```python
from build123d import *

# Parameters (mm, degrees)
F0_R     = 51.5
F1_DEPTH = 20
F2_R     = 49.925
F3_DEPTH = 17
F4_R     = 15.25
F5_DEPTH = 25
F8_R     = 10
F9_R     = 2


with BuildPart() as f1:
    # F0 (on Top) → F1 (new body)
    with BuildSketch(Plane.XY):
        Circle(F0_R)
    extrude(amount=F1_DEPTH)

    # F2 (on face) → F3 (cut)
    with BuildSketch(Plane.XY.offset(20)):
        Circle(F2_R)
    extrude(amount=-F3_DEPTH, mode=Mode.SUBTRACT)

    # F4 (on face) → F5 (cut)
    with BuildSketch(Plane(origin=(0, 0, 0), x_dir=(1, 0, 0), z_dir=(0, 0, -1))):
        Circle(F4_R)
    extrude(amount=-F5_DEPTH, mode=Mode.SUBTRACT)

    # F7: sweep along a path in F7_path
    with BuildLine(Plane(origin=(51.5, 0, 0), x_dir=(0, -1, 0), z_dir=(0, 0, -1))) as f7_path:
        CenterArc((0, 51.5), 51.5, 0, 360)
    # F6 (on Right) → F7 (sweep)
    with BuildSketch(Plane.YZ):
        Polygon((17.2497715373, 0.0302291046), (15.25, 0), (15.9, -43), (17.8997715373, -42.9697708954), align=None)
    sweep(path=f7_path.line)

    # F8
    f8_edges = [f1.edges().sort_by_distance(p)[0] for p in [
        (0, 17.250228, 0),
    ]]
    fillet(f8_edges, radius=F8_R)

    # F9
    f9_edges = [f1.edges().sort_by_distance(p)[0] for p in [
        (-49.925, 0, 3),
    ]]
    fillet(f9_edges, radius=F9_R)


solid = f1.part
```
Could you check a few things on this model? Use its own coordinates, in mm. A direction names the side the tool comes from. Round coordinates to 2 decimals unless told otherwise and drop trailing zeros. Loops run counter-clockwise (first coordinate to the right, second up) from the corner with the lowest first, then second, coordinate; pieces in that order, holes last. Notation, with made-up numbers: (46.25, 89) - (98.25, 89) arc R26 ccw to (98.25, 107) - close; hole circle Ø6 at (67, -7). An arc over 180 degrees is marked (long way). Answer as CSV lines item,"result".
1. We'd pull the mould along Z, two halves only. Please class faces 1 (the face through (-50, 4, 20)), 2 (the face through (22, -22, 0)), 3 (the face through (-10.82, -48.74, 12.6)), 4 (the face through (10.739, 14.005, -26.331)): +Z half, -Z half, draft (parallel to the pull), parting line (faces both ways), or undercut.
Filled in:
face 1,"+Z half"
face 2,"-Z half"
face 3,"draft"
face 4,"undercut"
2. On a 3-axis mill with a long thin cutter (end or side, diameter ignored), from which of +Z, -Z, +X, -X, +Y, -Y can I reach the whole of each face in a straight line? I mean faces 5 (the face through (-0.685, 15.564, -21.801)), 6 (the face through (-11.164, -50.275, 9.86)), 7 (the face through (-11, 11, 3)). Say none if no direction works.
Filled in:
face 5,"-Z"
face 6,"+Z, -Z"
face 7,"+Z"
3. I want a section at B-B on z = -6. List the corners of the cut face in (x, y) for me.
Filled in:
outline,"circle Ø36.47 at (0, 0); hole circle Ø30.68 at (0, 0)"
4. I want a section at A-A on z = 11. List the corners of the cut face in (x, y) for me (3 decimals), then the cut area to 3 significant figures.
Filled in:
outline,"circle Ø103 at (0, 0); hole circle Ø99.85 at (0, 0)"
area,"502 mm^2"
5. Please list where these lines run through material, in increasing order: line 1 along Y through (x, z) = (0, 16.5) (3 decimals); line 2 along Z through (x, y) = (-19.5, -29); line 3 along X through (y, z) = (-9.5, -24.5). Write a range as [from, to].
Filled in:
line 1,"y = [-51.5, -49.925], [49.925, 51.5]"
line 2,"z = [0, 3]"
line 3,"x = [-14.84, -12.4], [12.4, 14.84]"
6. For pin 1 Ø2 at (x, y) = (39, -26.5) entering from +Z; pin 2 Ø6 at (x, y) = (-24.5, 40) entering from -Z; pin 3 Ø3 at (y, z) = (-20.5, -15.5) entering from -X; pin 4 Ø1.5 at (y, z) = (-24.5, 3.5) entering from +X, each with a flat end and sliding along its axis, tell me the tip position at first contact or that it passes through.
Filled in:
pin 1,"stops at z = 3.01"
pin 2,"stops at z = 0"
pin 3,"passes through"
pin 4,"stops at x = 45.7"
